Could you check a few things on this model? Use its own coordinates, in mm. Give positions to 0.01 mm unless a question says otherwise; leave off trailing zeros.
(1) If I drill on probe 1 along Y at (x, z) = (0, -389); probe 2 along Y at (x, z) = (-5, -346); probe 3 along X at (y, z) = (10, -367), over which ranges is the centre line in solid material (lowest first)?
(2) Will these pins go through, and if not, where does the flat tip stop? pin 1 (4 mm diameter, centred on x = 7, y = -10.5, fed in from +Z); pin 2 (0.7 mm diameter, centred on y = 8.5, z = -265.5, fed in from -X).
(3) Imagine slicing it at A-A, the plane z = -155. State how many separate pieces and enclosed holes the cut face has, then the cut area to 3 significant figures.
Autodesk Inventor part; units mm, degrees
ref_plane "C1_XY" through (0, 0, 0) normal (0, 0, 1) x (1, 0, 0)
ref_plane "C1_YZ" through (0, 0, 0) normal (1, 0, 0) x (0, 1, 0)
ref_plane "C1_ZX" through (0, 0, 0) normal (0, 1, 0) x (0, 0, 1)
sketch "Sketch_1" plane through (0, 0, 0) normal (0, 0, 1) x (1, 0, 0)
  line L0 (-10, -7) -> (-8, -7)
  line L1 (-8, -7) -> (-8, -4)
  line L2 (-8, -4) -> (-7.0607, -4)
  line L3 (-7.0607, -4) -> (-4, -7.0607)
  line L4 (-4, -7.0607) -> (-4, -9.4804)
  line L5 (-4, -9.4804) -> (-3.7, -10)
  line L6 (-3.7, -10) -> (-4, -10.5196)
  line L7 (-4, -10.5196) -> (-4, -12.9393)
  line L8 (-4, -12.9393) -> (-7.0607, -16)
  line L9 (-7.0607, -16) -> (-8, -16)
  line L10 (-8, -16) -> (-8, -13)
  line L11 (-8, -13) -> (-10, -13)
  line L12 (-10, -13) -> (-10, -19)
  arc A0 (-10, -19) -> (-9, -20) centre (-9, -19) ccw
  line L13 (-9, -20) -> (-3, -20)
  line L14 (-3, -20) -> (-3, -18)
  line L15 (-3, -18) -> (-6, -18)
  line L16 (-6, -18) -> (-6, -17.0607)
  line L17 (-6, -17.0607) -> (-2.9393, -14)
  line L18 (-2.9393, -14) -> (-0.5196, -14)
  line L19 (-0.5196, -14) -> (0, -13.7)
  line L20 (0, -13.7) -> (0.5196, -14)
  line L21 (0.5196, -14) -> (2.9393, -14)
  line L22 (2.9393, -14) -> (6, -17.0607)
  line L23 (6, -17.0607) -> (6, -18)
  line L24 (6, -18) -> (3, -18)
  line L25 (3, -18) -> (3, -20)
  line L26 (3, -20) -> (9, -20)
  arc A1 (9, -20) -> (10, -19) centre (9, -19) ccw
  line L27 (10, -19) -> (10, -13)
  line L28 (10, -13) -> (8, -13)
  line L29 (8, -13) -> (8, -16)
  line L30 (8, -16) -> (7.0607, -16)
  line L31 (7.0607, -16) -> (4, -12.9393)
  line L32 (4, -12.9393) -> (4, -10.5196)
  line L33 (4, -10.5196) -> (3.7, -10)
  line L34 (3.7, -10) -> (4, -9.4804)
  line L35 (4, -9.4804) -> (4, -7.0607)
  line L36 (4, -7.0607) -> (7.0607, -4)
  line L37 (7.0607, -4) -> (8, -4)
  line L38 (8, -4) -> (8, -7)
  line L39 (8, -7) -> (10, -7)
  line L40 (10, -7) -> (10, 7)
  line L41 (10, 7) -> (8, 7)
  line L42 (8, 7) -> (8, 4)
  line L43 (8, 4) -> (7.0607, 4)
  line L44 (7.0607, 4) -> (4, 7.0607)
  line L45 (4, 7.0607) -> (4, 9.4804)
  line L46 (4, 9.4804) -> (3.7, 10)
  line L47 (3.7, 10) -> (4, 10.5196)
  line L48 (4, 10.5196) -> (4, 12.9393)
  line L49 (4, 12.9393) -> (7.0607, 16)
  line L50 (7.0607, 16) -> (8, 16)
  line L51 (8, 16) -> (8, 13)
  line L52 (8, 13) -> (10, 13)
  line L53 (10, 13) -> (10, 19)
  arc A2 (10, 19) -> (9, 20) centre (9, 19) ccw
  line L54 (9, 20) -> (3, 20)
  line L55 (3, 20) -> (3, 18)
  line L56 (3, 18) -> (6, 18)
  line L57 (6, 18) -> (6, 17.0607)
  line L58 (6, 17.0607) -> (2.9393, 14)
  line L59 (2.9393, 14) -> (0.5196, 14)
  line L60 (0.5196, 14) -> (0, 13.7)
  line L61 (0, 13.7) -> (-0.5196, 14)
  line L62 (-0.5196, 14) -> (-2.9393, 14)
  line L63 (-2.9393, 14) -> (-6, 17.0607)
  line L64 (-6, 17.0607) -> (-6, 18)
  line L65 (-6, 18) -> (-3, 18)
  line L66 (-3, 18) -> (-3, 20)
  line L67 (-3, 20) -> (-9, 20)
  arc A3 (-9, 20) -> (-10, 19) centre (-9, 19) ccw
  line L68 (-10, 19) -> (-10, 13)
  line L69 (-10, 13) -> (-8, 13)
  line L70 (-8, 13) -> (-8, 16)
  line L71 (-8, 16) -> (-7.0607, 16)
  line L72 (-7.0607, 16) -> (-4, 12.9393)
  line L73 (-4, 12.9393) -> (-4, 10.5196)
  line L74 (-4, 10.5196) -> (-3.7, 10)
  line L75 (-3.7, 10) -> (-4, 9.4804)
  line L76 (-4, 9.4804) -> (-4, 7.0607)
  line L77 (-4, 7.0607) -> (-7.0607, 4)
  line L78 (-7.0607, 4) -> (-8, 4)
  line L79 (-8, 4) -> (-8, 7)
  line L80 (-8, 7) -> (-10, 7)
  line L81 (-10, 7) -> (-10, -7)
  line L82 (-8, 1.7) -> (-8, -1.7)
  arc A4 (-8, -1.7) -> (-7.7, -2) centre (-7.7, -1.7) ccw
  line L83 (-7.7, -2) -> (-7.0636, -2)
  arc A5 (-6.8515, -2.0879) -> (-7.0636, -2) centre (-7.0636, -2.3) ccw
  line L84 (-6.8515, -2.0879) -> (-2.9393, -6)
  line L85 (-2.9393, -6) -> (2.9393, -6)
  line L86 (2.9393, -6) -> (6.8515, -2.0879)
  arc A6 (7.0636, -2) -> (6.8515, -2.0879) centre (7.0636, -2.3) ccw
  line L87 (7.0636, -2) -> (7.7, -2)
  arc A7 (7.7, -2) -> (8, -1.7) centre (7.7, -1.7) ccw
  line L88 (8, -1.7) -> (8, 1.7)
  arc A8 (8, 1.7) -> (7.7, 2) centre (7.7, 1.7) ccw
  line L89 (7.7, 2) -> (7.0636, 2)
  arc A9 (6.8515, 2.0879) -> (7.0636, 2) centre (7.0636, 2.3) ccw
  line L90 (6.8515, 2.0879) -> (2.9393, 6)
  line L91 (2.9393, 6) -> (-2.9393, 6)
  line L92 (-2.9393, 6) -> (-6.8515, 2.0879)
  arc A10 (-7.0636, 2) -> (-6.8515, 2.0879) centre (-7.0636, 2.3) ccw
  line L93 (-7.0636, 2) -> (-7.7, 2)
  arc A11 (-7.7, 2) -> (-8, 1.7) centre (-7.7, 1.7) ccw
extrude "Extrusion1" add sketch "Sketch_1" against normal blind 510
sketch "Sketch2" plane through (0, 0, -510) normal (0, 0, -1) x (-1, 0, 0)
  point P0 (0, 10)
hole "Hole1" at (0, 10, -510) direction (0, 0, 1) diameter 4.2 depth 510
pattern_linear "Rectangular Pattern1" count 2 spacing 20 along (0, -1, 0) of "Hole1"
ref_plane "C1_XY" through (0, 0, 0) normal (0, 0, 1) x (1, 0, 0)
ref_plane "C1_YZ" through (0, 0, 0) normal (1, 0, 0) x (0, 1, 0)
ref_plane "C1_ZX" through (0, 0, 0) normal (0, 1, 0) x (0, 0, 1)
properties part number "HFS5-2040-510"
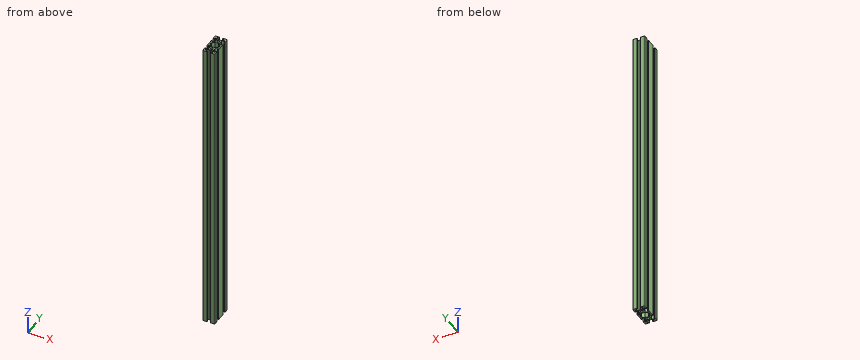
Answer block:
1. probe 1: y = -13.7 to -12.1, -7.9 to -6, 6 to 7.9, 12.1 to 13.7
1. probe 2: y = -20 to -18, -16.06 to -13.94, -6.06 to -3.94, 3.94 to 6.06, 13.94 to 16.06, 18 to 20
1. probe 3: x = -3.7 to -2.1, 2.1 to 3.7
2. pin 1: passes through
2. pin 2: stops at x = -4
3. separate pieces: 1
3. enclosed holes: 3
3. area: 324 mm2
